Job drawing, mm, ordinate dimensions from the low corner. One solid piece. Round coordinates to 2 decimals unless told otherwise and drop trailing zeros. Loops run counter-clockwise (first coordinate to the right, second up) from the corner with the lowest first, then second, coordinate; pieces in that order, holes last. Notation, with made-up numbers: M 55.25,-34.75 L 72.25,-34.75 A28 cw 72.25,-0.75 Z; hole C 56,78.25 d6. An arc over 180 degrees is marked long. Use a Markdown table: item, result. Add a question column.
(1) Band-saw the part on A-A, the plane x = 16.5. Write the cut outline in (y, z) (1 decimal).
(2) Band-saw the part on B-B, the plane y = 17. Write the cut outline in (x, z).
(3) Flat gauge pins, fed straight in: P1, Ø6, axis at x = 19.5, z = 1.5, coming from the +Y side (1 decimal); P2, Ø4, axis at x = 19.5, z = 8, coming from the -Y side. Where does each tip first touch, or does it go through?
(4) Band-saw the part on D-D, the plane z = 8. Write the cut outline in (x, y).
(5) Wall check: L1, parallel to Y at x = 15, z = 6; L2, parallel to X at y = 16.5, z = 1.25 (1 decimal). Give the ranges that are in metal, low to high.
(6) Band-saw the part on C-C, the plane x = 12.5. Write the cut outline in (y, z), and give its area (3 significant figures).
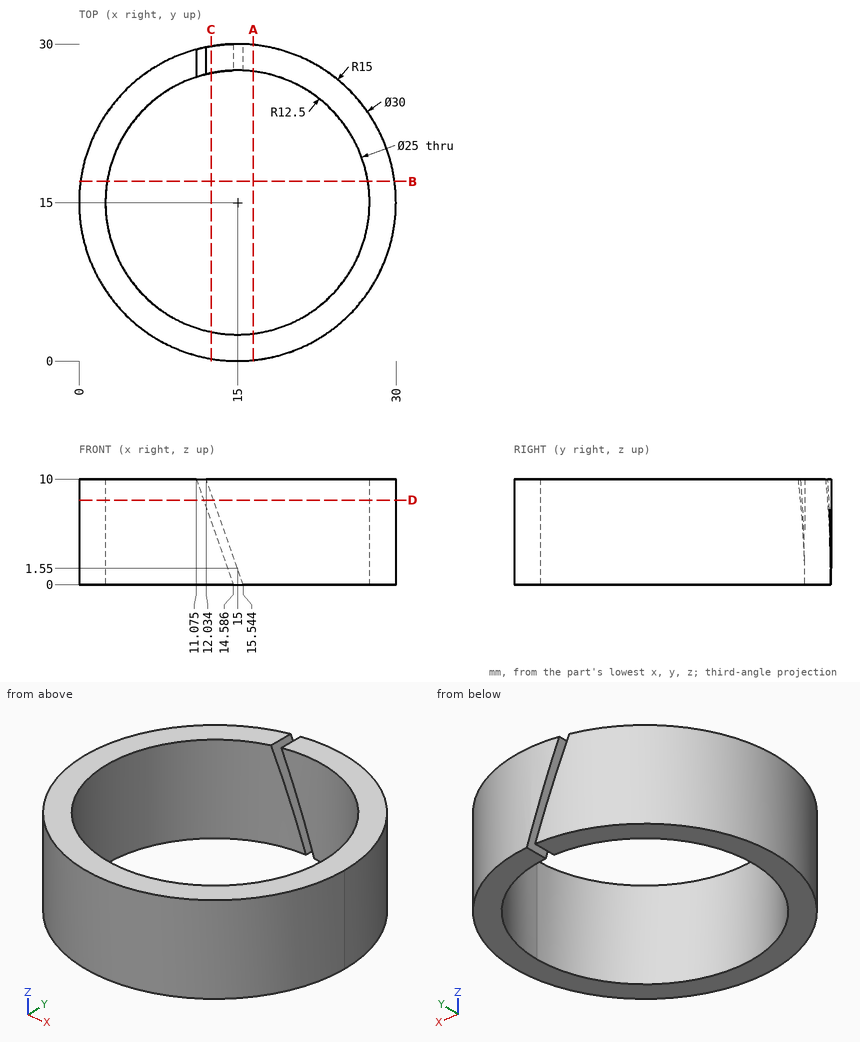
Return value:
| question | item | result |
|---|---|---|
| 1 | outline | M 0.1,0 L 2.6,0 L 2.6,10 L 0.1,10 Z; M 27.4,0 L 29.9,0 L 29.9,10 L 27.4,10 Z |
| 2 | outline | M 0.13,0 L 2.66,0 L 2.66,10 L 0.13,10 Z; M 27.34,0 L 29.87,0 L 29.87,10 L 27.34,10 Z |
| 3 | P1 | y = 29.9 |
| 3 | P2 | y = 0.21 |
| 4 | outline | M 11.78,27.08 L 11.78,29.65 A15 ccw long 12.74,29.83 L 12.74,27.29 A12.5 cw long Z |
| 5 | L1 | 0 to 2.5, 27.5 to 30 |
| 5 | L2 | 0.1 to 2.6, 27.4 to 29.9 |
| 6 | outline | M 0.21,0 L 2.75,0 L 2.75,10 L 0.21,10 Z; M 27.25,0 L 29.79,0 L 29.79,5.94 L 27.25,5.94 Z; M 27.25,8.67 L 29.79,8.67 L 29.79,10 L 27.25,10 Z |
| 6 | area | 43.9 mm^2 |
